from build123d import *

# Parameters (mm, degrees)
SKETCH2_R                                         = 16.256
BOSS_EXTRUDE1_DEPTH                               = 3.175
SKETCH3_W                                         = 63.5
SKETCH3_H                                         = 4.445
BOSS_EXTRUDE2_DEPTH                               = 3.175
CSK_FOR_0_FLAT_HEAD_MACHINE_SCREW_100_D           = 3.000000096
CSK_FOR_0_FLAT_HEAD_MACHINE_SCREW_100_CSINK_D     = 3.0226
CSK_FOR_0_FLAT_HEAD_MACHINE_SCREW_100_CSINK_ANGLE = 100
SKETCH6_R                                         = 1.27
CUT_EXTRUDE1_DEPTH                                = 6.35


with BuildPart() as part:
    # Sketch2 → Boss-Extrude1 (new body, symmetric)
    with BuildSketch(Plane(origin=(0, 0, 0), x_dir=(0, 0, -1), z_dir=(1, 0, 0))):
        Polygon((-20.32, 4.445), (20.32, 4.445), (31.75, 4.445), (31.75, 0), (-31.75, 0), (-31.75, 4.445), align=None)
        with BuildLine():
            ThreePointArc((-20.32, 20.85), (0, 41.17), (20.32, 20.85))
            Line((20.32, 20.85), (20.32, 4.445))
            Line((20.32, 4.445), (-20.32, 4.445))
            Line((-20.32, 4.445), (-20.32, 20.85))
        make_face()
        with Locations((0, 20.85)):
            Circle(SKETCH2_R, mode=Mode.SUBTRACT)
    extrude(amount=BOSS_EXTRUDE1_DEPTH, both=True)

    # Sketch3 → Boss-Extrude2 (add)
    with BuildSketch(Plane(origin=(3.175, 0, 0), x_dir=(0, 0, -1), z_dir=(1, 0, 0))):
        with Locations((0, 2.2225)):
            Rectangle(SKETCH3_W, SKETCH3_H)
    extrude(amount=BOSS_EXTRUDE2_DEPTH)

    # CSK for #0 Flat Head Machine Screw (100)1 (through all)
    with Locations(Plane(origin=(0, 0, -20.32), x_dir=(-1, 0, 0), z_dir=(0, 0, -1))):
        with Locations((0, 20.85)):
            CounterSinkHole(CSK_FOR_0_FLAT_HEAD_MACHINE_SCREW_100_D / 2, CSK_FOR_0_FLAT_HEAD_MACHINE_SCREW_100_CSINK_D / 2, counter_sink_angle=CSK_FOR_0_FLAT_HEAD_MACHINE_SCREW_100_CSINK_ANGLE)

    # Sketch6 → Cut-Extrude1 (cut)
    with BuildSketch(Plane(origin=(0, 4.445, 0), x_dir=(1, 0, 0), z_dir=(0, 1, 0))):
        with Locations((1.5875, -26.67)):
            Circle(SKETCH6_R)
    cut_extrude1 = extrude(amount=-CUT_EXTRUDE1_DEPTH, mode=Mode.SUBTRACT)

    # Mirror2: Cut-Extrude1 across plane
    add(cut_extrude1.mirror(Plane.XY), mode=Mode.SUBTRACT)


solid = part.part
Model file for the job. Use its own axes, mm. A direction names the side the tool comes from. Give positions to 0.01 mm unless a question says otherwise; leave off trailing zeros. Loops run counter-clockwise (first coordinate to the right, second up) from the corner with the lowest first, then second, coordinate; pieces in that order, holes last.
1) Tool access for faces 4 (the cylindrical face through (0.044, 41.165, 0.447)), 5 (the flat face through (3.175, 32.4, -12.1)), 6 (the flat face through (0, 13, 20.32)), 7 (the flat face through (4, 4.445, 0)), 8 (the flat face through (0, 13, -20.32)): list every direction of +Z, -Z, +X, -X, +Y, -Y with a clear straight run to the whole face (end or side of a thin tool).
2) Wall check: line 1 (Z direction, x = 1.75, y = 20.85); line 2 (Y direction, x = 5.5, z = -7) (3 decimals); line 3 (X direction, y = 6.5, z = 16.5) (3 decimals). Give the ranges that are in metal, low to high.
3) Saw through at C-C (x = 5.5). Write the cut outline in (y, z) (3 decimals), plus the area to 3 significant figures.
4) Saw through at B-B (y = 14). Write the cut outline in (x, z) (3 decimals).
5) Pull direction Z, two halves, no side cores. Call faces 1 (the cylindrical face through (1.42, 2.25, -25.41)), 2 (the flat face through (2, 2, -31.75)), 3 (the flat face through (-3.175, 4, 0)): +Z half, -Z half, draft (parallel to the pull), parting line (faces both ways), or undercut.
6) Flat gauge pins, fed straight in: pin 1 Ø1.9 at (x, y) = (-0.5, 10.5) entering from -Z; pin 2 Ø3 at (x, z) = (3.5, 15.5) entering from +Y; pin 3 Ø1.9 at (x, y) = (0, 12) entering from +Z. Where does each tip first touch, or does it go through?
7) Saw through at D-D (z = 9). Write the cut outline in (x, y) (3 decimals), plus the area to 3 significant figures.
Answer block:
1. face 4: +X, -X, +Y
1. face 5: +Z, -Z, +X, +Y
1. face 6: +Z, +X, -X, +Y
1. face 7: +X, +Y
1. face 8: -Z, +X, -X, +Y
2. line 1: z = -20.32 to -16.26, 16.26 to 20.32
2. line 2: y = 0 to 4.445
2. line 3: x = -3.175 to 3.175
3. outline: (0, -31.75) - (4.445, -31.75) - (4.445, 31.75) - (0, 31.75) - close
3. area: 282 mm2
4. outline: (-3.175, -20.32) - (3.175, -20.32) - (3.175, -14.742) - (-3.175, -14.742) - close; (-3.175, 14.742) - (3.175, 14.742) - (3.175, 20.32) - (-3.175, 20.32) - close
5. face 1: undercut
5. face 2: -Z half
5. face 3: draft
6. pin 1: stops at z = -20.32
6. pin 2: stops at y = 35.54
6. pin 3: stops at z = 20.32
7. outline: (-3.175, 0) - (6.35, 0) - (6.35, 4.445) - (3.175, 4.445) - (3.175, 7.313) - (-3.175, 7.313) - close; (-3.175, 34.387) - (3.175, 34.387) - (3.175, 39.068) - (-3.175, 39.068) - close
7. area: 90.3 mm2
